```python
from build123d import *

# Parameters (mm, degrees)
PAD043_DEPTH = 23.5
SKETCH047_R  = 11.4
PAD044_DEPTH = 2
SKETCH048_R  = 2.5
PAD045_DEPTH = 20


with BuildPart() as part:
    # Sketch046 → Pad043 (new body)
    with BuildSketch(Plane.XY):
        Polygon((-15.5, 21), (-21, 15.5), (-21, -15.5), (-15.5, -21), (15.5, -21), (21, -15.5), (21, 15.5), (15.5, 21), align=None)
    extrude(amount=-PAD043_DEPTH)

    # Sketch047 (on Face9 of Pad043) → Pad044 (join)
    with BuildSketch(Plane.XY):
        Circle(SKETCH047_R)
    extrude(amount=PAD044_DEPTH)

    # Sketch048 (on Face12 of Pad044) → Pad045 (join)
    with BuildSketch(Plane.XY.offset(2)):
        Circle(SKETCH048_R)
    extrude(amount=PAD045_DEPTH)


solid = part.part
```
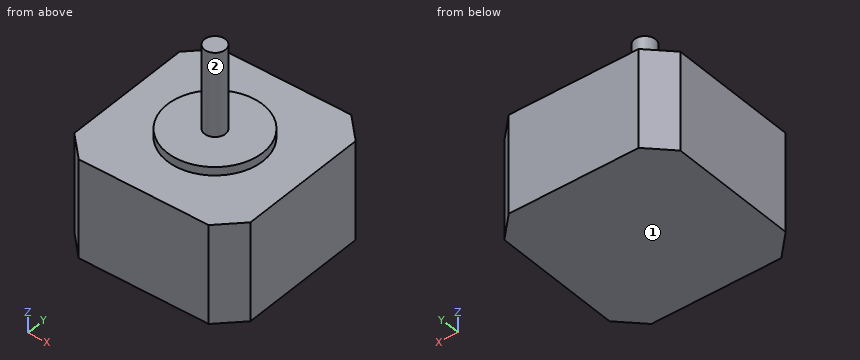
Input: part model. Units: mm. Frame: model coordinates. Face numbers are marked on the shaded views. A direction names the side the tool comes from. Round coordinates to 2 decimals unless told otherwise and drop trailing zeros. Loops run counter-clockwise (first coordinate to the right, second up) from the corner with the lowest first, then second, coordinate; pieces in that order, holes last.
1) Material intervals for line 1 (Z direction, x = 9.5, y = -1); line 2 (Z direction, x = -8.5, y = -8.5); line 3 (X direction, y = 19, z = -1), sorted ascending.
Ans:
line 1: z = -23.5 to 2
line 2: z = -23.5 to 0
line 3: x = -17.5 to 17.5
2) Pin query (flat end, axial travel): pin 1 (10 mm diameter, centred on x = -11.5, z = 16.5, fed in from -Y); pin 2 (6 mm diameter, centred on x = -8, y = -1, fed in from +Z); pin 3 (25 mm diameter, centred on x = 0.5, y = 5.5, fed in from +Z); pin 4 (10 mm diameter, centred on x = 4.5, z = 15.5, fed in from +Y). Return the tip coordinate at first contact, or that it passes through.
Ans:
pin 1: passes through
pin 2: stops at z = 2
pin 3: stops at z = 22
pin 4: stops at y = 2.5
3) Section query A-A on x = 0. Return the cut outline in (y, z), plus the area to 3 significant figures.
Ans:
outline: (-21, -23.5) - (21, -23.5) - (21, 0) - (11.4, 0) - (11.4, 2) - (2.5, 2) - (2.5, 22) - (-2.5, 22) - (-2.5, 2) - (-11.4, 2) - (-11.4, 0) - (-21, 0) - close
area: 1,130 mm2
4) Section query D-D on y = 17. Return the cut outline in (x, z), plus the area to 4 significant figures.
Ans:
outline: (-19.5, -23.5) - (19.5, -23.5) - (19.5, 0) - (-19.5, 0) - close
area: 916.5 mm2
5) Section query C-C on x = 4.5. Return the cut outline in (y, z).
Ans:
outline: (-21, -23.5) - (21, -23.5) - (21, 0) - (10.47, 0) - (10.47, 2) - (-10.47, 2) - (-10.47, 0) - (-21, 0) - close
6) Set-up query: the marked faces 1 and 2. Return all of +Z, -Z, +X, -X, +Y, -Y with unobstructed straight access to the full face (end or side cutting, diameter ignored); none if empty.
Ans:
face 1: -Z, +X, -X, +Y, -Y
face 2: +Z
